Geometry: see drawing. Coordinates: mm, zero at the bounding-box minimum. Give positions to 0.01 mm unless a question says otherwise; leave off trailing zeros. Loops run counter-clockwise (first coordinate to the right, second up) from the corner with the lowest first, then second, coordinate; pieces in that order, holes last. Notation, with made-up numbers: (77.5, 61) -> (132.5, 61) arc R9 cw to (132.5, 74) -> close; hole circle Ø8 at (-23, 51.25). An arc over 180 degrees is marked (long way). Answer in a Markdown table with one row per item. Add a question column.
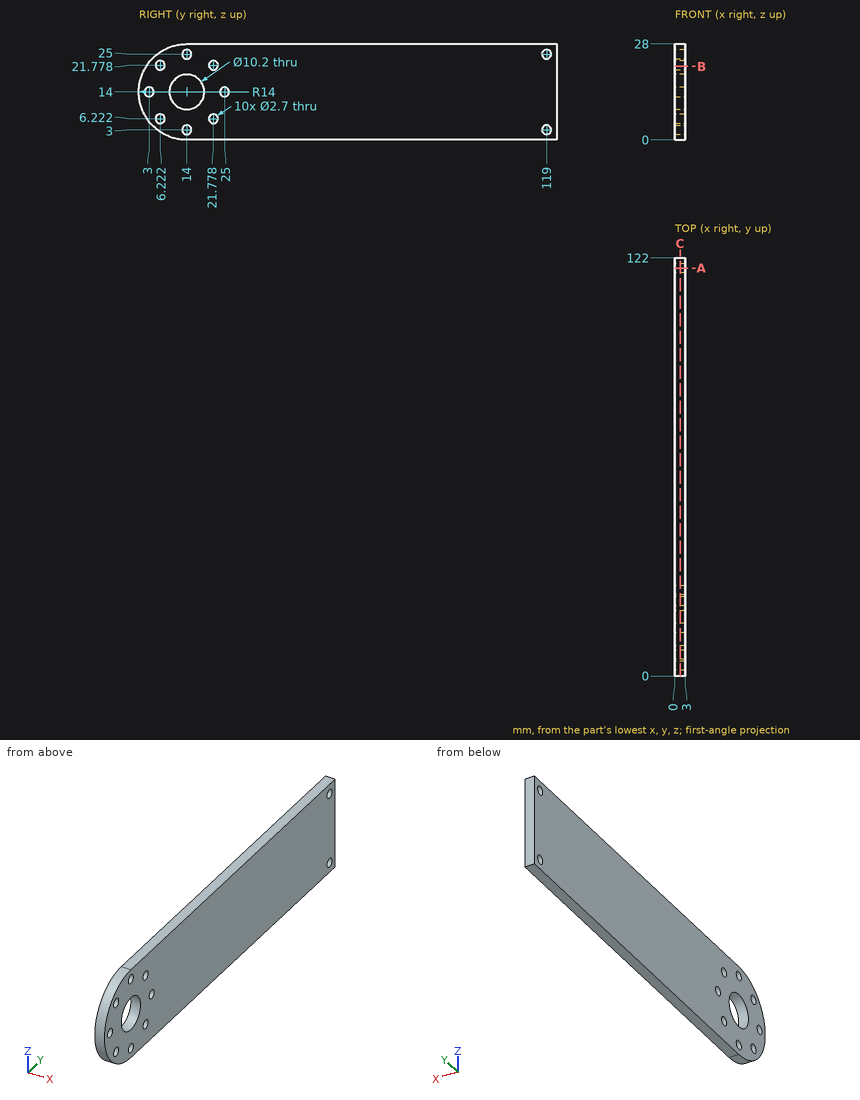
1) Section B-B on z = 21.5. Output: boundary loops of the cut face in (x, y), and give its area (3 significant figures).
2) Material intervals for line 1 along Y through (x, z) = (1.85, 14); line 2 along Z through (x, y) = (1.95, 119); line 3 along Y through (x, z) = (1.55, 6.75), sorted ascending.
3) Section C-C on x = 1.55. State how many separate pieces and enclosed holes the cut face has, and give its area (3 significant figures).
4) Section A-A on y = 119. Output: boundary loops of the cut face in (x, z).
Working result:
| question | item | result |
|---|---|---|
| 1 | outline | (0, 2.18) -> (3, 2.18) -> (3, 4.9) -> (0, 4.9) -> close; (0, 7.54) -> (3, 7.54) -> (3, 20.46) -> (0, 20.46) -> close; (0, 23.1) -> (3, 23.1) -> (3, 122) -> (0, 122) -> close |
| 1 | area | 344 mm2 |
| 2 | line 1 | y = 0 to 1.65, 4.35 to 8.9, 19.1 to 23.65, 26.35 to 122 |
| 2 | line 2 | z = 0 to 1.65, 4.35 to 23.65, 26.35 to 28 |
| 2 | line 3 | y = 2.02 to 4.98, 7.46 to 20.54, 23.02 to 122 |
| 3 | separate pieces | 1 |
| 3 | enclosed holes | 11 |
| 3 | area | 3,190 mm2 |
| 4 | outline | (0, 0) -> (3, 0) -> (3, 1.65) -> (0, 1.65) -> close; (0, 4.35) -> (3, 4.35) -> (3, 23.65) -> (0, 23.65) -> close; (0, 26.35) -> (3, 26.35) -> (3, 28) -> (0, 28) -> close |
